The model under review builds one solid part; all positions refer to its coordinate system, in mm. Face numbers are marked on the shaded views. A direction names the side the tool comes from. Round coordinates to 2 decimals unless told otherwise and drop trailing zeros. Order: outer loops, then holes, each group sorted by start corner. A loop starts at its lowest first (then second) coordinate and runs counter-clockwise, first axis right, second up. Notation, with made-up numbers: (75, -30) - (121, -30) arc R10 ccw to (121, -16) - close; hole circle Ø6 at (65.5, -10). An arc over 180 degrees is marked (long way). One line per question, with ' | ' between items. Start each with the question number.
Item 1: Tool access review of the marked faces 4, 5 and 6: name each direction out of +Z, -Z, +X, -X, +Y, -Y from which nothing blocks a thin tool from reaching the whole face with its end or side.
Item 2: Add section D-D on y = 6.5. State the section outline as (x, z) points.
Item 3: Add section A-A on y = 8.5. State the section outline as (x, z) points.
Item 4: Add section B-B on z = 0. State the section outline as (x, y) points, and give its area (3 significant figures).
Item 5: Draft analysis for pull direction Z (two halves, no side actions). For the marked faces 1, 2 and 3, state which applies: +Z half, -Z half, draft (parallel to the pull), parting line (faces both ways), or undercut.
Item 6: Insertion check: pin 1 Ø1 at (y, z) = (13, -1) entering from +X; pin 2 Ø6 at (y, z) = (8, 1) entering from -X; pin 3 Ø3 at (x, y) = (-4.5, 10.5) entering from +Z. Each pin has a flat end and moves straight along its axis. Give the tip position at first contact, or say it passes through.
Item 7: For L1, parallel to X at y = 0.65, z = 0; L2, parallel to Z at x = -18, y = 0.35; L3, parallel to X at y = 5.25, z = 2.75, list the stretches that pass through material, from the lowest coordinate up. Write a range as [from, to].
Item 8: Add section C-C on x = -3. State the section outline as (y, z) points, and give its area (3 significant figures).
from build123d import *

# Parameters (mm, degrees)
SKETCH_1_R          = 1.5
EXTRUDE_1_DEPTH     = 1
SKETCH_3_W          = 29
SKETCH_3_H          = 12.5
EXTRUDE_2_DEPTH     = 14
SKETCH_4_W          = 10
SKETCH_4_H          = 6
EXTRUDE_3_DEPTH     = 8
SKETCH_5_W          = 29
SKETCH_5_H          = 2.25
CUT_EXTRUDE_1_DEPTH = 6
SKETCH_6_W          = 29
SKETCH_6_H          = 12.5
SKETCH_6_W_2        = 27
SKETCH_6_H_2        = 7
CUT_EXTRUDE_2_DEPTH = 2
SKETCH_7_W          = 4
SKETCH_7_H          = 7
CUT_EXTRUDE_3_DEPTH = 2


with BuildPart() as part:
    # 草图1 → 凸台-拉伸1 (new body)
    with BuildSketch(Plane(origin=(0, 0, 0), x_dir=(1, 0, 0), z_dir=(0, 1, 0))):
        with BuildLine():
            Line((-18, -3.5), (18, -3.5))
            ThreePointArc((18, -3.5), (21.5, 0), (18, 3.5))
            Line((18, 3.5), (-18, 3.5))
            ThreePointArc((-18, 3.5), (-21.5, 0), (-18, -3.5))
        make_face()
        with Locations((-18, 0)):
            Circle(SKETCH_1_R, mode=Mode.SUBTRACT)
        with Locations((18, 0)):
            Circle(SKETCH_1_R, mode=Mode.SUBTRACT)
    extrude(amount=EXTRUDE_1_DEPTH)

    # 草图3 → 凸台-拉伸2 (add)
    with BuildSketch(Plane.XZ):
        Rectangle(SKETCH_3_W, SKETCH_3_H)
    extrude(amount=-EXTRUDE_2_DEPTH)

    # 草图4 → 凸台-拉伸3 (add)
    with BuildSketch(Plane(origin=(0, 0, -6.25), x_dir=(-1, 0, 0), z_dir=(0, 0, -1))):
        with Locations((0, 7)):
            Rectangle(SKETCH_4_W, SKETCH_4_H)
    extrude(amount=EXTRUDE_3_DEPTH)

    # 草图5 → 切除-拉伸1 (cut)
    with BuildSketch(Plane(origin=(0, 14, 0), x_dir=(1, 0, 0), z_dir=(0, 1, 0))):
        with Locations((0, 5.125)):
            Rectangle(SKETCH_5_W, SKETCH_5_H)
        with Locations((0, -5.125)):
            Rectangle(SKETCH_5_W, SKETCH_5_H)
    extrude(amount=-CUT_EXTRUDE_1_DEPTH, mode=Mode.SUBTRACT)

    # 草图6 → 切除-拉伸2 (cut)
    with BuildSketch(Plane(origin=(0, 14, 0), x_dir=(1, 0, 0), z_dir=(0, 1, 0))):
        Rectangle(SKETCH_6_W, SKETCH_6_H)
        Rectangle(SKETCH_6_W_2, SKETCH_6_H_2, mode=Mode.SUBTRACT)
    extrude(amount=-CUT_EXTRUDE_2_DEPTH, mode=Mode.SUBTRACT)

    # 草图7 → 切除-拉伸3 (cut)
    with BuildSketch(Plane(origin=(0, 14, 0), x_dir=(1, 0, 0), z_dir=(0, 1, 0))):
        with Locations((-4.5, 0)):
            Rectangle(SKETCH_7_W, SKETCH_7_H)
    extrude(amount=-CUT_EXTRUDE_3_DEPTH, mode=Mode.SUBTRACT)


solid = part.part
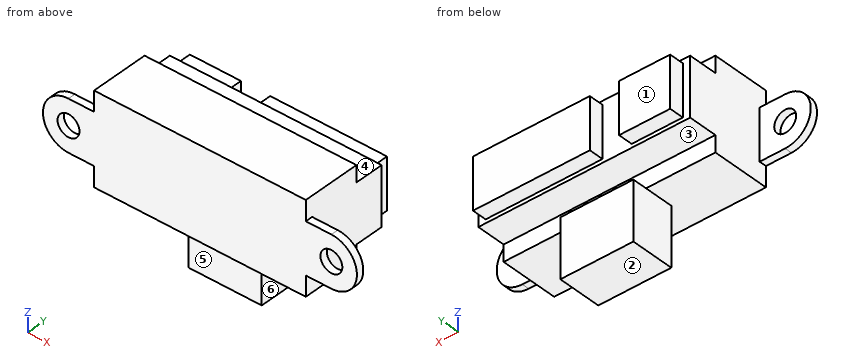
Determined:
1) face 4: +Z, +X, -X, +Y | face 5: -Z, +X, -X, -Y | face 6: -Z, +X, +Y, -Y
2) outline: (-14.5, -6.25) - (-5, -6.25) - (-5, -14.25) - (5, -14.25) - (5, -6.25) - (14.5, -6.25) - (14.5, 6.25) - (-14.5, 6.25) - close
3) outline: (-14.5, -4) - (14.5, -4) - (14.5, 4) - (-14.5, 4) - close; (-5, -14.25) - (5, -14.25) - (5, -6.25) - (-5, -6.25) - close
4) outline: (-21.5, 0) - (-19.5, 0) - (-19.5, 1) - (-21.5, 1) - close; (-16.5, 0) - (16.5, 0) - (16.5, 1) - (14.5, 1) - (14.5, 12) - (13.5, 12) - (13.5, 14) - (-2.5, 14) - (-2.5, 12) - (-6.5, 12) - (-6.5, 14) - (-13.5, 14) - (-13.5, 12) - (-14.5, 12) - (-14.5, 1) - (-16.5, 1) - close; (19.5, 0) - (21.5, 0) - (21.5, 1) - (19.5, 1) - close | area: 402 mm2
5) face 1: draft | face 2: -Z half | face 3: undercut
6) pin 1: x = 13.5 | pin 2: x = -14.5 | pin 3: z = 4
7) L1: [-21.5, -19.5], [-16.5, 16.5], [19.5, 21.5] | L2: [-3.5, -1.5], [1.5, 3.5] | L3: [-14.5, 14.5]
8) outline: (0, -6.25) - (4, -6.25) - (4, -14.25) - (10, -14.25) - (10, -6.25) - (8, -6.25) - (8, -4) - (12, -4) - (12, 4) - (8, 4) - (8, 6.25) - (0, 6.25) - close | area: 180 mm2
